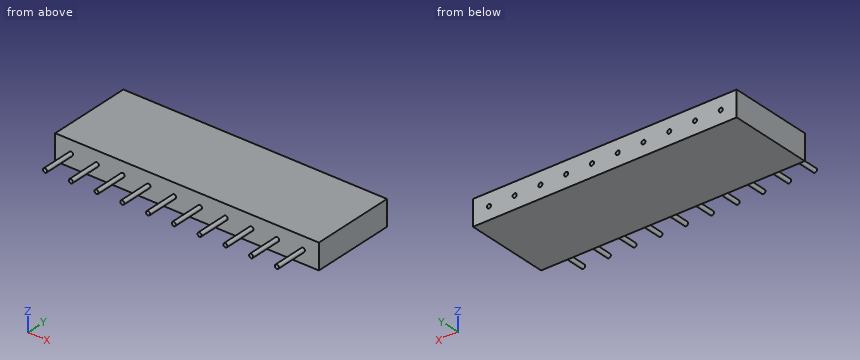
```python
from build123d import *

# Parameters (mm, degrees)
SKETCH1_W           = 26
SKETCH1_H           = 2.5
BOSS_EXTRUDE1_DEPTH = 8.35
SKETCH2_R           = 0.2
CUT_EXTRUDE1_DEPTH  = 3
SKETCH3_R           = 0.2
BOSS_EXTRUDE2_DEPTH = 3.2
LPATTERN1_COUNT     = 10
LPATTERN1_PITCH     = 2.54


with BuildPart() as part:
    # Sketch1 → Boss-Extrude1 (new body)
    with BuildSketch(Plane(origin=(0, 0, 0), x_dir=(1, 0, 0), z_dir=(0, 1, 0))):
        Rectangle(SKETCH1_W, SKETCH1_H)
    extrude(amount=BOSS_EXTRUDE1_DEPTH)

    # Sketch2 → Cut-Extrude1 (cut)
    with BuildSketch(Plane(origin=(0, 8.35, 0), x_dir=(1, 0, 0), z_dir=(0, 1, 0))):
        with Locations((-11.43, 0)):
            Circle(SKETCH2_R)
    cut_extrude1 = extrude(amount=-CUT_EXTRUDE1_DEPTH, mode=Mode.SUBTRACT)

    # Sketch3 → Boss-Extrude2 (add)
    with BuildSketch(Plane.XZ):
        with Locations((-11.43, 0)):
            Circle(SKETCH3_R)
    boss_extrude2 = extrude(amount=BOSS_EXTRUDE2_DEPTH)

    # LPattern1: Cut-Extrude1, Boss-Extrude2 ×10
    with Locations(*[(i * LPATTERN1_PITCH, 0, 0) for i in range(1, LPATTERN1_COUNT)]):
        add(cut_extrude1, mode=Mode.SUBTRACT)
        add(boss_extrude2)


solid = part.part
```
Here's how the part is built. I have some questions about the finished solid (model axes, mm). Coordinates: 2 decimals unless noted, no trailing zeros. Write each loop counter-clockwise with the first axis right and the second up, starting at its lowest first coordinate (ties: lowest second). Pieces come first, ordered by that corner, then holes. Notation, with made-up numbers: (-29, 76) -> (26, 76) arc R33 ccw to (26, 109) -> close; hole circle Ø1 at (4.5, -26.5). An arc over 180 degrees is marked (long way). Use a Markdown table: item, result. Add a question column.
(1) If we section it at C-C, the plane x = 4.5: Write out the boundary of the cut face in (y, z), and give its area (3 significant figures).
(2) If we section it at B-B, the plane z = 0.7: Write out the boundary of the cut face in (x, y).
(3) If we section it at A-A, the plane y = 6.75: State how many separate pieces and enclosed holes the cut face has, and give its area (3 significant figures).
(4) Please list where these lines run through material, in increasing order: line 1 (Z direction, x = -6.35, y = 6.3); line 2 (Y direction, x = 5.75, z = -0.7).
Outcome:
| question | item | result |
|---|---|---|
| 1 | outline | (0, -1.25) -> (8.35, -1.25) -> (8.35, 1.25) -> (0, 1.25) -> close |
| 1 | area | 20.9 mm^2 |
| 2 | outline | (-13, 0) -> (13, 0) -> (13, 8.35) -> (-13, 8.35) -> close |
| 3 | separate pieces | 1 |
| 3 | enclosed holes | 10 |
| 3 | area | 63.7 mm^2 |
| 4 | line 1 | z = -1.25 to -0.2, 0.2 to 1.25 |
| 4 | line 2 | y = 0 to 8.35 |
